```python
from build123d import *

# Parameters (mm, degrees)
BOSS_EXTRUDE1_START     = 1057.012834
BOSS_EXTRUDE1_DEPTH     = 50.8
CUT_EXTRUDE1_DEPTH      = 1125.4772971
CUT_EXTRUDE1_DEPTH_BACK = 1125.4772971
SKETCH2_R               = 3.302
BOSS_EXTRUDE2_START     = 1057.012834
BOSS_EXTRUDE2_DEPTH     = 6.35
BOSS_EXTRUDE3_START     = 1101.462834
BOSS_EXTRUDE3_DEPTH     = 6.35


with BuildPart() as part:
    # Sketch1 → Boss-Extrude1 (new body)
    with BuildSketch(Plane.XY.offset(BOSS_EXTRUDE1_START)):
        Polygon((152.527062484, 81.531574554), (152.527062484, 87.881574554), (130.604002291, 87.881574554), (130.604002291, 118.048344881), (124.254002291, 118.048344881), (124.254002291, 81.531574554), align=None)
    extrude(amount=BOSS_EXTRUDE1_DEPTH)

    # Sketch2 → Cut-Extrude1 (cut, two sides: drawn at the far end of the back side and taken through both)
    with BuildSketch(Plane(origin=(0, 0, 0), x_dir=(1, 0, 0), z_dir=(0, 1, 0)).offset(-CUT_EXTRUDE1_DEPTH_BACK)):
        with Locations(Location((146.050062484, -1068.125334154, 0), (0, 0, 90))):
            Circle(SKETCH2_R)
    extrude(amount=CUT_EXTRUDE1_DEPTH + CUT_EXTRUDE1_DEPTH_BACK, mode=Mode.SUBTRACT)

    # Sketch3 → Boss-Extrude2 (add)
    with BuildSketch(Plane.XY.offset(BOSS_EXTRUDE2_START)):
        Polygon((130.604002291, 118.048344881), (152.527062484, 87.881574554), (130.604002291, 87.881574554), align=None)
    extrude(amount=BOSS_EXTRUDE2_DEPTH)

    # Sketch3<2> → Boss-Extrude3 (add)
    with BuildSketch(Plane.XY.offset(BOSS_EXTRUDE3_START)):
        Polygon((130.604002291, 118.048344881), (152.527062484, 87.881574554), (130.604002291, 87.881574554), align=None)
    extrude(amount=BOSS_EXTRUDE3_DEPTH)


solid = part.part
```
Source: CAD feature listing. Evaluate the final solid. Frame: model axes, mm. A direction names the side the tool comes from. Round coordinates to 2 decimals unless told otherwise and drop trailing zeros. Loops run counter-clockwise (first coordinate to the right, second up) from the corner with the lowest first, then second, coordinate; pieces in that order, holes last. Notation, with made-up numbers: M 8.5,16.25 L 59.5,16.25 A5 ccw 59.5,21.25 Z; hole C -6,-9.75 d11. An arc over 180 degrees is marked long. Use a Markdown table: item, result. Add a question column.
1. Ray query, line 1 along Z through (x, y) = (138.75, 93); line 2 along X through (y, z) = (92, 1074); line 3 along Y through (x, z) = (141.75, 1076). Return the intervals inside material, ascending. Write a range as [from, to].
2. Cut plane A-A, the plane z = 1066. Output: boundary loops of the cut face in (x, y).
3. Contact query for flat-ended pins moving along their axis: pin 1 (12 mm diameter, centred on x = 146.5, z = 1099.5, fed in from +Y); pin 2 (1.5 mm diameter, centred on x = 143.5, z = 1085.5, fed in from +Y); pin 3 (1 mm diameter, centred on y = 110.5, z = 1100.5, fed in from +X). Output: stop coordinate, or through.
4. Cut plane D-D, the plane y = 114. Output: boundary loops of the cut face in (x, z).
5. Cut plane C-C, the plane z = 1080.5. Output: boundary loops of the cut face in (x, y), and give its area (3 significant figures).
6. Cut plane B-B, the plane x = 150.5. Output: boundary loops of the cut face in (y, z), and give its area (3 significant figures).
7. Set-up query: faces 1 (the flat face through (141.41, 103.18, 1104.59)), 2 (the flat face through (137, 96, 1063.363)). Return all of +Z, -Z, +X, -X, +Y, -Y with unobstructed straight access to the full face (end or side cutting, diameter ignored); none if empty.
Solution:
| question | item | result |
|---|---|---|
| 1 | line 1 | z = [1057.01, 1063.36], [1101.46, 1107.81] |
| 1 | line 2 | x = [124.25, 130.6] |
| 1 | line 3 | y = [81.53, 87.88] |
| 2 | outline | M 124.25,81.53 L 143.52,81.53 L 143.52,87.88 L 130.6,87.88 L 130.6,118.05 L 124.25,118.05 Z; M 148.58,81.53 L 152.53,81.53 L 152.53,87.88 L 148.58,87.88 Z |
| 3 | pin 1 | stops at y = 103.98 |
| 3 | pin 2 | stops at y = 87.88 |
| 3 | pin 3 | stops at x = 130.6 |
| 4 | outline | M 124.25,1057.01 L 133.55,1057.01 L 133.55,1063.36 L 130.6,1063.36 L 130.6,1101.46 L 133.55,1101.46 L 133.55,1107.81 L 124.25,1107.81 Z |
| 5 | outline | M 124.25,81.53 L 152.53,81.53 L 152.53,87.88 L 130.6,87.88 L 130.6,118.05 L 124.25,118.05 Z |
| 5 | area | 371 mm2 |
| 6 | outline | M 81.53,1057.01 L 90.67,1057.01 L 90.67,1063.36 L 87.88,1063.36 L 87.88,1101.46 L 90.67,1101.46 L 90.67,1107.81 L 81.53,1107.81 Z |
| 6 | area | 358 mm2 |
| 7 | face 1 | +Z, -Z, +X, +Y |
| 7 | face 2 | +X, +Y |
